```python
from build123d import *

# Parameters (mm, degrees)
F0_W     = 140
F0_H     = 140
F1_DEPTH = 12
F2_R     = 30
F3_DEPTH = 275
F4_R     = 20
F5_DEPTH = 275.001


with BuildPart() as f1:
    # F0 (on Top) → F1 (new body)
    with BuildSketch(Plane.XY):
        Rectangle(F0_W, F0_H)
    extrude(amount=-F1_DEPTH)

    # F2 (on face) → F3 (join)
    with BuildSketch(Plane.XY):
        Circle(F2_R)
    extrude(amount=-F3_DEPTH)

    # F4 (on face) → F5 (cut, through all)
    with BuildSketch(Plane(origin=(0, 0, -275), x_dir=(1, 0, 0), z_dir=(0, 0, -1))):
        Circle(F4_R)
    extrude(amount=-F5_DEPTH, mode=Mode.SUBTRACT)


solid = f1.part
```
Geometry: final body of the model. Coordinates: model frame, mm. A direction names the side the tool comes from. Coordinates: 2 decimals unless noted, no trailing zeros. Order: outer loops, then holes, each group sorted by start corner. A loop starts at its lowest first (then second) coordinate and runs counter-clockwise, first axis right, second up. Notation, with made-up numbers: (12.25, -33.75) - (48.25, -33.75) arc R18 ccw to (48.25, -26.75) - close; hole circle Ø2 at (36, 36.25). An arc over 180 degrees is marked (long way). Return JSON: item names as keys, results as strings. Group by question number.
1. Pin query (flat end, axial travel): pin 1 (12 mm diameter, centred on y = -21.5, z = -158, fed in from +X); pin 2 (2 mm diameter, centred on y = 7, z = -33, fed in from +X); pin 3 (1.5 mm diameter, centred on x = 26.5, z = -195.5, fed in from +Y). Return the tip coordinate at first contact, or that it passes through.
2. Cut plane C-C (x = 24). Output: boundary loops of the cut face in (y, z), plus the area to 3 significant figures.
3. Set-up query: faces 5 (the face through (-1, 32, -12)), 6 (the face through (-70, -1, -6)). Return all of +Z, -Z, +X, -X, +Y, -Y with unobstructed straight access to the full face (end or side cutting, diameter ignored); none if empty.
4. Cut plane D-D (z = -258). Output: boundary loops of the cut face in (x, y), plus the area to 3 significant figures.
5. Material intervals for line 1 along Y through (x, z) = (0, -169); line 2 along Z through (x, y) = (8, -33.5); line 3 along Y through (x, z) = (-5, -36), sorted ascending. Write a range as [from, to].
6. Cut plane A-A (x = 0). Output: boundary loops of the cut face in (y, z), plus the area to 3 significant figures.
7. Pull-direction query (X, two-part tool) for faces 1 (the face through (-29.97, 1.32, -141.66)), 2 (the face through (70, -1, -6)), 3 (the face through (-4.336, 19.524, -139.425)), 4 (the face through (-1, -70, -6)); classes: pulls with the +X half, pulls with the -X half, needs draft (parallel to the pull), parting line crosses it, or undercut.
Resolved:
{
 "1": {"pin 1": "stops at x = 25.69", "pin 2": "stops at x = 29.39", "pin 3": "stops at y = 15.39"},
 "2": {"outline": "(-70, -12) - (-18, -12) - (-18, -275) - (18, -275) - (18, -12) - (70, -12) - (70, 0) - (-70, 0) - close", "area": "11,100 mm²"},
 "3": {"face 5": "-Z", "face 6": "+Z, -Z, -X, +Y, -Y"},
 "4": {"outline": "circle Ø60 at (0, 0); hole circle Ø40 at (0, 0)", "area": "1,570 mm²"},
 "5": {"line 1": "y = [-30, -20], [20, 30]", "line 2": "z = [-12, 0]", "line 3": "y = [-29.58, -19.36], [19.36, 29.58]"},
 "6": {"outline": "(-70, -12) - (-30, -12) - (-30, -275) - (-20, -275) - (-20, 0) - (-70, 0) - close; (20, -275) - (30, -275) - (30, -12) - (70, -12) - (70, 0) - (20, 0) - close", "area": "6,460 mm²"},
 "7": {"face 1": "parting line crosses it", "face 2": "pulls with the +X half", "face 3": "undercut", "face 4": "needs draft"}
}
